Autodesk Inventor part; units mm, degrees
ref_plane "YZ Plane" through (0, 0, 0) normal (1, 0, 0) x (0, 1, 0)
ref_plane "XZ Plane" through (0, 0, 0) normal (0, 1, 0) x (-1, 0, 0)
ref_plane "XY Plane" through (0, 0, 0) normal (0, 0, 1) x (1, 0, 0)
sketch "Sketch1" plane through (0, 0, 0) normal (0, 0, 1) x (1, 0, 0)
  line L0 (0, 0) -> (48, 0)
  line L1 (48, 0) -> (48, 48)
  line L2 (48, 48) -> (0, 48)
  line L3 (0, 48) -> (0, 0)
  dimension "d0" = 48
  dimension "d1" = 48
extrude "Extrusion1" add sketch "Sketch1" along normal blind 15
sketch "Sketch2" plane through (0, 0, 15) normal (0, 0, 1) x (1, 0, 0)
  line L0 (6, 6) -> (42, 6)
  line L1 (42, 6) -> (42, 42)
  line L2 (42, 42) -> (6, 42)
  line L3 (6, 42) -> (6, 6)
  point P0 (0, 0)
  dimension "d6" = 36
  dimension "d7" = 36
extrude "Extrusion2" cut sketch "Sketch2" against normal blind 11
chamfer "Chamfer1" distance 4 angle 45 4 edges at (42, 24, 15) (24, 42, 15) (6, 24, 15) (24, 6, 15)
sketch "Sketch3" plane through (0, 0, 4) normal (0, 0, 1) x (1, 0, 0)
  line L0 (0, 0) -> (24, 0)
  line L1 (0, 24) -> (0, 0)
  line L2 (46, 46) -> (2, 46)
  line L3 (26.6, 24) -> (26.6, 24.8)
  line L4 (26.6, 24.8) -> (30.2, 24.8)
  line L5 (30.2, 24.8) -> (30.2, 23.2)
  line L6 (30.2, 23.2) -> (26.6, 23.2)
  line L7 (24, 21.4) -> (24.8, 21.4)
  line L8 (24.8, 21.4) -> (24.8, 17.8)
  line L9 (24.8, 17.8) -> (23.2, 17.8)
  line L10 (23.2, 17.8) -> (23.2, 21.4)
  line L11 (21.4, 23.2) -> (17.8, 23.2)
  line L12 (17.8, 23.2) -> (17.8, 24.8)
  line L13 (17.8, 24.8) -> (21.4, 24.8)
  line L14 (24, 26.6) -> (24.8, 26.6)
  line L15 (24.8, 26.6) -> (24.8, 30.2)
  line L16 (24.8, 30.2) -> (23.2, 30.2)
  line L17 (23.2, 30.2) -> (23.2, 26.6)
  line L18 (48, 48) -> (0, 48)
  line L19 (0, 48) -> (0, 0)
  circle A0 centre (38.1421, 31.0711) radius 1.25
  circle A1 centre (16.9289, 9.8579) radius 1.25
  line L20 (21.4, 23.2) -> (21.4, 24.8)
  line L21 (23.2, 26.6) -> (24, 26.6)
  line L22 (26.6, 23.2) -> (26.6, 24)
  line L23 (23.2, 21.4) -> (24, 21.4)
  circle A2 centre (26.6, 21.4) radius 1.25
  circle A3 centre (21.4, 26.6) radius 1.25
  circle A4 centre (26.6, 26.6) radius 1.25
  circle A5 centre (21.4, 21.4) radius 1.25
  line L24 (24, 24) -> (30.2, 24)
  circle A6 centre (30.2, 30.2) radius 1.25
  circle A7 centre (17.8, 30.2) radius 1.25
  circle A8 centre (17.8, 17.8) radius 1.25
  circle A9 centre (30.2, 17.8) radius 1.25
  circle A10 centre (9.8579, 9.8579) radius 1.25
  circle A11 centre (38.1421, 38.1421) radius 1.25
  point P0 (48, 0)
  dimension "d21" = 0.8
  dimension "d22" = 3.6
  dimension "d23" = 1.6
  dimension "d25" = 3.6
  dimension "d26" = 1.6
  dimension "d27" = 3.6
  dimension "d28" = 1.6
  dimension "d30" = 1.6
  dimension "d62" = 2.5
  dimension "d63" = 2.5
  dimension "d64" = 2.5
  dimension "d65" = 2.5
  dimension "d66" = 2.5
  dimension "d67" = 2.5
extrude "Extrusion4" cut sketch "Sketch3" against normal blind 5 contours A0 | A1 | A6 | A7 | A8 | A9
properties part number "one-square"
Build history of the part. All positions in model axes, mm. A direction names the side the tool comes from. Coordinates: 2 decimals unless noted, no trailing zeros. Order: outer loops, then holes, each group sorted by start corner. A loop starts at its lowest first (then second) coordinate and runs counter-clockwise, first axis right, second up.
Item 1: Saw through at D-D on x = 43. List the corners of the cut face in (y, z), then the cut area to 3 significant figures.
Filled in:
outline: (0, 0) - (48, 0) - (48, 15) - (46, 15) - (43, 12) - (5, 12) - (2, 15) - (0, 15) - close
area: 597 mm2
Item 2: Tool access for faces 1 (the cylindrical face through (37.98, 32.31, 2.03)), 2 (the flat face through (24, 4, 13)): list every direction of +Z, -Z, +X, -X, +Y, -Y with a clear straight run to the whole face (end or side of a thin tool).
Filled in:
face 1: +Z, -Z
face 2: +Z
Item 3: Drill centre lines: L1, parallel to Y at x = 30.2, z = 1.9; L2, parallel to Y at x = 17, z = 7.25. Where is each one in solid material? Low to high.
Filled in:
L1: y = 0 to 16.55, 19.05 to 28.95, 31.45 to 48
L2: y = 0 to 6, 42 to 48
Item 4: Saw through at C-C on z = 9.75. List the corners of the cut face in (x, y).
Filled in:
outline: (0, 0) - (48, 0) - (48, 48) - (0, 48) - close; hole (6, 6) - (42, 6) - (42, 42) - (6, 42) - close
Item 5: Drop flat-ended pins along their axis: pin 1 Ø3 at (x, y) = (30.2, 30.2) entering from -Z; pin 2 Ø3 at (x, y) = (30.2, 17.8) entering from +Z; pin 3 Ø3 at (x, y) = (6, 32.5) entering from +Z. Give the stop position or say it passes through.
Filled in:
pin 1: stops at z = 0
pin 2: stops at z = 4
pin 3: stops at z = 12.5
Item 6: Mould opens along X. For faces 3 (the flat face through (24, 42, 8)), 4 (the flat face through (44, 24, 13)), 5 (the flat face through (24, 48, 7)), 6 (the flat face through (48, 24, 7)) say: released by +X, released by -X, zero draft, split by the parting line, or undercut.
Filled in:
face 3: undercut
face 4: undercut
face 5: zero draft
face 6: released by +X
Item 7: Saw through at A-A on y = 17.8. List the corners of the cut face in (x, z), then the cut area to 3 significant figures.
Filled in:
outline: (0, 0) - (16.55, 0) - (16.55, 4) - (6, 4) - (6, 11) - (2, 15) - (0, 15) - close; (19.05, 0) - (28.95, 0) - (28.95, 4) - (19.05, 4) - close; (31.45, 0) - (48, 0) - (48, 15) - (46, 15) - (42, 11) - (42, 4) - (31.45, 4) - close
area: 288 mm2
